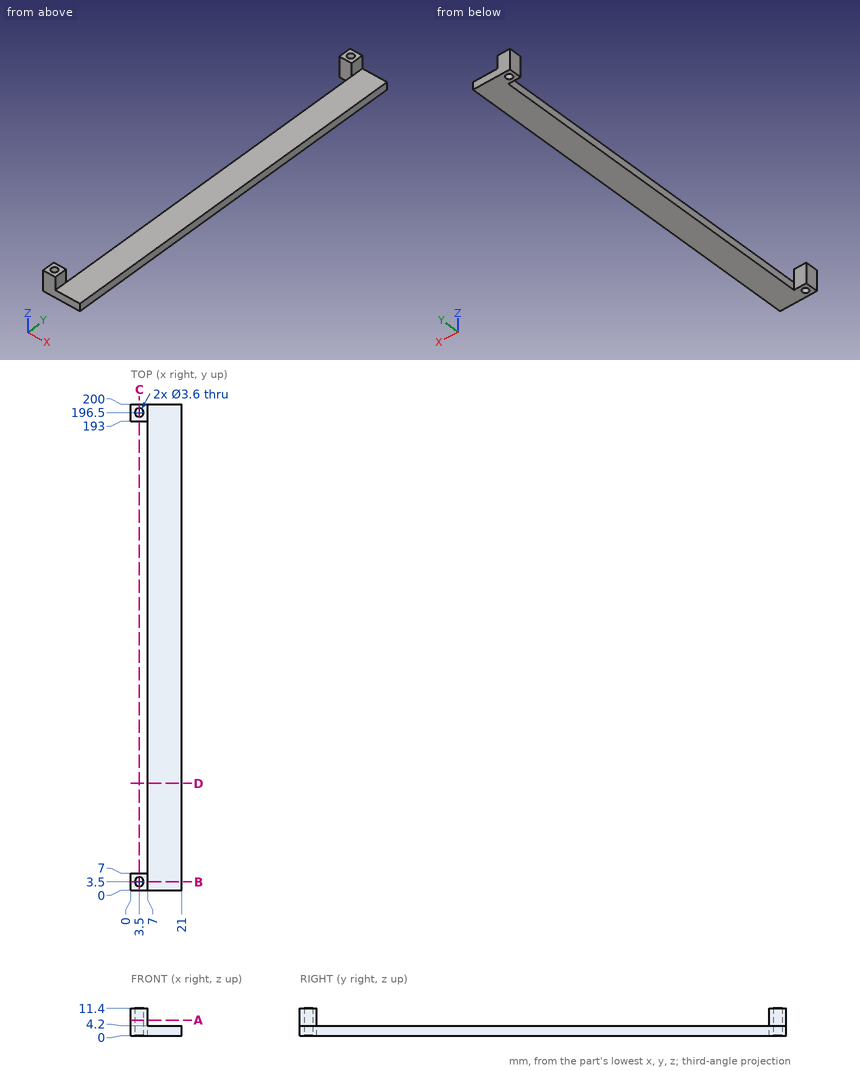
Here's the drawing with two shaded views (mm, measured from the low corner). I have some questions. Coordinates: 2 decimals unless noted, no trailing zeros. Write each loop counter-clockwise with the first axis right and the second up, starting at its lowest first coordinate (ties: lowest second). Pieces come first, ordered by that corner, then holes. Notation, with made-up numbers: (3, 37) -> (53, 37) arc R7 ccw to (53, 42) -> close; hole circle Ø11 at (16, -9.5). An arc over 180 degrees is marked (long way). Use a Markdown table: item, result. Add a question column.
(1) If we section it at C-C, the plane x = 3.5: Write out the boundary of the cut face in (y, z), and give its area (3 significant figures).
(2) Please list where these lines run through material, in increasing order: line 1 (Y direction, x = 3.5, z = 6.5); line 2 (Y direction, x = 5.75, z = 7); line 3 (Y direction, x = 3, z = 8.25).
(3) I'm going to push flat-ended pins straight in: P1, Ø6, axis at x = 16.5, y = 48.5, coming from the +Z side; P2, Ø2, axis at y = 4, z = 8, coming from the +X side; P3, Ø3, axis at x = 3.5, y = 3.5, coming from the -Z side; P4, Ø4.5, axis at y = 61, z = 2.5, coming from the -X side. Where does each tip first touch, or does it pass through?
(4) If we section it at D-D, the plane y = 44: Write out the boundary of the cut face in (x, z), and give its area (3 significant figures).
(5) If we section it at A-A, the plane z = 6.5: Write out the boundary of the cut face in (x, y).
(6) If we section it at B-B, the plane y = 3.5: Write out the boundary of the cut face in (x, z), and give its area (3 significant figures).
Outcome:
| question | item | result |
|---|---|---|
| 1 | outline | (0, 0) -> (1.7, 0) -> (1.7, 11.4) -> (0, 11.4) -> close; (5.3, 0) -> (7, 0) -> (7, 11.4) -> (5.3, 11.4) -> close; (193, 0) -> (194.7, 0) -> (194.7, 11.4) -> (193, 11.4) -> close; (198.3, 0) -> (200, 0) -> (200, 11.4) -> (198.3, 11.4) -> close |
| 1 | area | 77.5 mm^2 |
| 2 | line 1 | y = 0 to 1.7, 5.3 to 7, 193 to 194.7, 198.3 to 200 |
| 2 | line 2 | y = 0 to 7, 193 to 200 |
| 2 | line 3 | y = 0 to 1.77, 5.23 to 7, 193 to 194.77, 198.23 to 200 |
| 3 | P1 | stops at z = 4.2 |
| 3 | P2 | stops at x = 7 |
| 3 | P3 | passes through |
| 3 | P4 | stops at x = 7 |
| 4 | outline | (7, 0) -> (21, 0) -> (21, 4.2) -> (7, 4.2) -> close |
| 4 | area | 58.8 mm^2 |
| 5 | outline | (0, 0) -> (7, 0) -> (7, 7) -> (0, 7) -> close; (0, 193) -> (7, 193) -> (7, 200) -> (0, 200) -> close; hole circle Ø3.6 at (3.5, 3.5); hole circle Ø3.6 at (3.5, 196.5) |
| 6 | outline | (0, 0) -> (1.7, 0) -> (1.7, 11.4) -> (0, 11.4) -> close; (5.3, 0) -> (21, 0) -> (21, 4.2) -> (7, 4.2) -> (7, 11.4) -> (5.3, 11.4) -> close |
| 6 | area | 97.6 mm^2 |
